from build123d import *

# Parameters (mm, degrees)
SKETCH3_R                            = 5
BOSS_EXTRUDE1_DEPTH                  = 6
SKETCH4_R                            = 4.5
BOSS_EXTRUDE2_DEPTH                  = 10
BOSS_EXTRUDE2_DRAFT                  = -8
MIRROR1_COPY_1_SKETCH_R              = 4.5
MIRROR1_COPY_1_DEPTH                 = 10
MIRROR1_COPY_1_DRAFT                 = -8
SKETCH5_R                            = 3
BOSS_EXTRUDE3_DEPTH                  = 25
BOSS_EXTRUDE3_DIRECTION_2_REACH      = 22.244
BOSS_EXTRUDE3_DIRECTION_2_END_RADIUS = 5
SKETCH6_R                            = 5
BOSS_EXTRUDE4_DEPTH                  = 10
F_5_0MM_DOWEL_HOLE1_D                = 5
F_5_0MM_DOWEL_HOLE1_DEPTH            = 10
F_5_0MM_DOWEL_HOLE1_TIP              = 1.502151548
SKETCH9_R                            = 5.905408347
BOSS_EXTRUDE5_DEPTH                  = 1.5
BOSS_EXTRUDE5_TAPER                  = 63
FILLET1_R                            = 1
FILLET2_R                            = 0.5


with BuildPart() as part:
    # Sketch3 → Boss-Extrude1 (new, symmetric)
    with BuildSketch(Plane(origin=(0, 0, 0), x_dir=(0, 0, -1), z_dir=(1, 0, 0))):
        with Locations((0, 40)):
            Circle(SKETCH3_R)
    extrude(amount=BOSS_EXTRUDE1_DEPTH, both=True)


with BuildPart() as boss_extrude2_tool:
    # Sketch4 → Boss-Extrude2 (with draft: the straight prism first)
    with BuildSketch(Plane(origin=(6, 0, 0), x_dir=(0, 0, -1), z_dir=(1, 0, 0))):
        with Locations((0, 40)):
            Circle(SKETCH4_R)
    extrude(amount=BOSS_EXTRUDE2_DEPTH)
    # Boss-Extrude2: the draft: its side faces are tilted about the plane it starts from
    boss_extrude2_sides = [boss_extrude2_tool.faces().sort_by_distance(p)[0] for p in [
        (11, 40, 4.5),
    ]]
    draft(boss_extrude2_sides, Plane(origin=(6, 0, 0), x_dir=(0, 0, -1), z_dir=(1, 0, 0)), BOSS_EXTRUDE2_DRAFT)


with BuildPart() as part_1:
    add(part.part)

    # Boss-Extrude2: add boss_extrude2_tool
    add(boss_extrude2_tool.part)


with BuildPart() as mirror1_copy_1_tool:
    # Mirror1 copy 1 sketch → Mirror1 copy 1 (with draft: the straight prism first)
    with BuildSketch(Plane(origin=(-6, 0, 0), x_dir=(0, 0, -1), z_dir=(-1, 0, 0))):
        with Locations((0, -40)):
            Circle(MIRROR1_COPY_1_SKETCH_R)
    extrude(amount=MIRROR1_COPY_1_DEPTH)
    # Mirror1 copy 1: the draft: its side faces are tilted about the plane it starts from
    mirror1_copy_1_sides = [mirror1_copy_1_tool.faces().sort_by_distance(p)[0] for p in [
        (-11, 40, 4.5),
    ]]
    draft(mirror1_copy_1_sides, Plane(origin=(-6, 0, 0), x_dir=(0, 0, -1), z_dir=(-1, 0, 0)), MIRROR1_COPY_1_DRAFT)


with BuildPart() as part_2:
    add(part_1.part)

    # Mirror1 copy 1: add mirror1_copy_1_tool
    add(mirror1_copy_1_tool.part)

    # Sketch5 → Boss-Extrude3 (add)
    with BuildSketch(Plane(origin=(0, 35, 0), x_dir=(-1, 0, 0), z_dir=(0, -1, 0))):
        with Locations(Location((0, 0, 0), (0, 0, 270))):
            Circle(SKETCH5_R)
    extrude(amount=BOSS_EXTRUDE3_DEPTH)

    # Boss-Extrude3 direction 2: up to this cylinder (the profile starts outside it)
    boss_extrude3_direction_2_end = Plane(origin=(0, 40, 0), z_dir=(-1, 0, 0)) * Cylinder(BOSS_EXTRUDE3_DIRECTION_2_END_RADIUS, 55.488, mode=Mode.PRIVATE)
    # Sketch5 → Boss-Extrude3 direction 2 (add, up to the surface)
    with BuildSketch(Plane(origin=(0, 35, 0), x_dir=(-1, 0, 0), z_dir=(0, -1, 0)), mode=Mode.PRIVATE) as boss_extrude3_direction_2_sk1:
        with Locations(Location((0, 0, 0), (0, 0, 270))):
            Circle(SKETCH5_R)
    boss_extrude3_direction_2_tool1 = extrude(boss_extrude3_direction_2_sk1.sketch, amount=-BOSS_EXTRUDE3_DIRECTION_2_REACH, mode=Mode.PRIVATE) - boss_extrude3_direction_2_end
    add(boss_extrude3_direction_2_tool1.solids().sort_by_distance((0, 35, 0))[0])
    add(boss_extrude3_direction_2_tool1.solids().sort_by_distance((0, 35, 0))[1])

    # Sketch6 → Boss-Extrude4 (add)
    with BuildSketch(Plane.XZ.offset(-10)):
        with Locations(Location((0, 0, 0), (0, 0, 270))):
            Circle(SKETCH6_R)
    extrude(amount=BOSS_EXTRUDE4_DEPTH)

    # Ø5.0mm Dowel Hole1
    with Locations(Plane(origin=(0, 0, 0), x_dir=(-1, 0, 0), z_dir=(0, -1, 0))):
        with Locations((0, 0)):
            Hole(F_5_0MM_DOWEL_HOLE1_D / 2, depth=F_5_0MM_DOWEL_HOLE1_DEPTH)
            with Locations((0, 0, -(F_5_0MM_DOWEL_HOLE1_DEPTH + F_5_0MM_DOWEL_HOLE1_TIP / 2))):  # 118° drill point
                Cone(0, F_5_0MM_DOWEL_HOLE1_D / 2, F_5_0MM_DOWEL_HOLE1_TIP, mode=Mode.SUBTRACT)

    # Sketch9 → Boss-Extrude5 (add)
    with BuildSketch(Plane(origin=(16, 0, 0), x_dir=(0, 0, -1), z_dir=(1, 0, 0))):
        with Locations((0, 40)):
            Circle(SKETCH9_R)
    boss_extrude5 = extrude(amount=BOSS_EXTRUDE5_DEPTH, taper=BOSS_EXTRUDE5_TAPER)

    # Mirror2: Boss-Extrude5 across plane
    add(boss_extrude5.mirror(Plane(origin=(0, 0, 0), x_dir=(0, 0, 1), z_dir=(1, 0, 0))))

    # Fillet1
    fillet1_edges = [part_2.edges().sort_by_distance(p)[0] for p in [
        (3.000000007, 34.999999994, -1e-09),
    ]]
    fillet(fillet1_edges, radius=FILLET1_R)

    # Fillet2
    fillet2_edges = [part_2.edges().sort_by_distance(p)[0] for p in [
        (-16, 40, 5.905408347),
        (16, 40, 5.905408347),
    ]]
    fillet(fillet2_edges, radius=FILLET2_R)


solid = part_2.part
Verification items for the finished model (mm, model axes). A direction names the side the tool comes from. Give positions to 0.01 mm unless a question says otherwise; leave off trailing zeros. Write each loop counter-clockwise with the first axis right and the second up, starting at its lowest first coordinate (ties: lowest second). Pieces come first, ordered by that corner, then holes. Notation, with made-up numbers: (26, 0.25) - (52, 0.25) arc R26 ccw to (52, 26.25) - close; hole circle Ø5 at (83, 46.25). An arc over 180 degrees is marked (long way). Answer as CSV lines item,"result". Start each with the question number.
1. Sectioned sample at B-B (z = 4.5). Count the separate pieces of the cut face and the enclosed holes in it, then the cut area to 3 significant figures.
2. Sectioned sample at C-C (y = 29.5). Record the boundary of the cut face in (x, z).
3. Sectioned sample at A-A (y = 5). Record the boundary of the cut face in (x, z), then the cut area to 3 significant figures.
4. Thickness scan on line 1 (X direction, y = 4, z = -1.5); line 2 (X direction, y = 15.5, z = -0.25); line 3 (X direction, y = 8, z = -1). Record the ranges inside material, lowest first.
5. Draft check along Y on faces 1 (the face through (0.084, 44.957, 0.651)), 2 (the face through (17.5, 40, 0)), 3 (the face through (-2, 0, -2)). Enter one of: pulls with the +Y half, pulls with the -Y half, needs draft (parallel to the pull), parting line crosses it, or undercut.
6. Depth check by flat-ended pin: pin 1 (4.5 mm diameter, centred on x = 0, z = 0, fed in from +Y); pin 2 (2 mm diameter, centred on x = -12, z = 1.5, fed in from -Y); pin 3 (4 mm diameter, centred on y = 27, z = 2, fed in from -X). Enter the tip coordinate at first touch or a pass-through.
7. Set-up check for faces 4 (the face through (-4.88, 5.07, 1.08)), 5 (the face through (9.68, 35.55, -2.32)), 6 (the face through (-17.5, 40, 0)): record each of +Z, -Z, +X, -X, +Y, -Y from which the full face is reachable in a straight line by a thin tool's end or side.
8. Sectioned sample at D-D (x = 10). Record the boundary of the cut face in (y, z), then the cut area to 3 significant figures.
Derived:
1,separate pieces,"4"
1,enclosed holes,"0"
1,area,"202 mm²"
2,outline,"circle Ø6 at (0, 0)"
3,outline,"circle Ø10 at (0, 0); hole circle Ø5 at (0, 0)"
3,area,"58.9 mm²"
4,line 1,"-4.77 to -2, 2 to 4.77"
4,line 2,"-2.99 to 2.99"
4,line 3,"-4.9 to -2.29, 2.29 to 4.9"
5,face 1,"undercut"
5,face 2,"needs draft"
5,face 3,"pulls with the -Y half"
6,pin 1,"y = 45"
6,pin 2,"y = 34.62"
6,pin 3,"x = -3"
7,face 4,"-Y"
7,face 5,"none"
7,face 6,"+Z, -Z, -X, +Y, -Y"
8,outline,"circle Ø10.12 at (40, 0)"
8,area,"80.5 mm²"
